Input: part model. Units: mm. Frame: model coordinates. Face numbers are marked on the shaded views. A direction names the side the tool comes from. Coordinates: 2 decimals unless noted, no trailing zeros. Write each loop counter-clockwise with the first axis right and the second up, starting at its lowest first coordinate (ties: lowest second). Pieces come first, ordered by that corner, then holes.
1) Section query D-D (x = -35). Output: boundary loops of the cut face in (y, z).
2) Draft query along X for the marked faces 4, 5, 6 and 7. Return one class per face: pulls with the +X half, pulls with the -X half, needs draft (parallel to the pull), parting line crosses it, or undercut.
3) Section query A-A (z = -18). Output: boundary loops of the cut face in (x, y).
4) Line query: L1, parallel to Z at x = -35, y = -13; L2, parallel to Y at x = -32, z = -43; L3, parallel to X at y = -11.5, z = -32. Output: solid intervals per line, ascending.
5) Pin query (flat end, axial travel): pin 1 Ø12 at (y, z) = (11.5, -42.5) entering from -X; pin 2 Ø20 at (x, y) = (-25.5, -6) entering from -Z; pin 3 Ø4 at (x, y) = (2.5, -11) entering from -Z. Return the tip coordinate at first contact, or that it passes through.
6) Set-up query: the marked faces 1, 2 and 3. Return all of +Z, -Z, +X, -X, +Y, -Y with unobstructed straight access to the full face (end or side cutting, diameter ignored); none if empty.
7) Section query B-B (x = 24). Output: boundary loops of the cut face in (y, z).
8) Section query C-C (z = -39). Output: boundary loops of the cut face in (x, y), then the cut area to 3 significant figures.
from build123d import *

# Parameters (mm, degrees)
SKETCH2_R           = 20
BOSS_EXTRUDE1_DEPTH = 8
CUT_EXTRUDE2_DEPTH  = 65.319514924
BOSS_EXTRUDE2_DEPTH = 12
SKETCH6_R           = 10
CUT_EXTRUDE3_DEPTH  = 91.647669578
FILLET2_R           = 1.2
FILLET3_R           = 1.2


with BuildPart() as part:
    # Sketch2 → Boss-Extrude1 (new, symmetric)
    with BuildSketch(Plane.XY):
        with BuildLine():
            Line((39, 20), (-59, 20))
            Line((-59, 20), (-59, -20))
            Line((-59, -20), (39, -20))
            ThreePointArc((39, -20), (19, 0), (39, 20))
        make_face()
        with Locations((39, 0)):
            Circle(SKETCH2_R)
    extrude(amount=BOSS_EXTRUDE1_DEPTH, both=True)

    # Sketch3 → Cut-Extrude2 (cut, through all)
    with BuildSketch(Plane.XY.offset(8)):
        with BuildLine():
            ThreePointArc((14.284953176, 0), (11.941807426, 5.656854249), (6.284953176, 8))
            Line((6.284953176, 8), (6.284953176, -8))
            ThreePointArc((6.284953176, -8), (11.941807426, -5.656854249), (14.284953176, 0))
        make_face()
        with BuildLine():
            Line((6.284953176, -8), (6.284953176, 8))
            ThreePointArc((6.284953176, 8), (-1.715046824, 0), (6.284953176, -8))
        make_face()
        with BuildLine():
            Line((30.284953176, 8), (6.284953176, 8))
            ThreePointArc((6.284953176, 8), (11.941807426, 5.656854249), (14.284953176, 0))
            ThreePointArc((14.284953176, 0), (11.941807426, -5.656854249), (6.284953176, -8))
            Line((6.284953176, -8), (30.284953176, -8))
            ThreePointArc((30.284953176, -8), (22.284953176, 0), (30.284953176, 8))
        make_face()
        with BuildLine():
            ThreePointArc((38.284953176, 0), (35.941807426, 5.656854249), (30.284953176, 8))
            Line((30.284953176, 8), (30.284953176, -8))
            ThreePointArc((30.284953176, -8), (35.941807426, -5.656854249), (38.284953176, 0))
        make_face()
        with BuildLine():
            Line((30.284953176, -8), (30.284953176, 8))
            ThreePointArc((30.284953176, 8), (22.284953176, 0), (30.284953176, -8))
        make_face()
    extrude(amount=-CUT_EXTRUDE2_DEPTH, mode=Mode.SUBTRACT)

    # Sketch5 → Boss-Extrude2 (add)
    with BuildSketch(Plane(origin=(0, 20, 0), x_dir=(1, 0, 0), z_dir=(0, 1, 0))):
        with BuildLine():
            ThreePointArc((-59, 32), (-51.970562748, 15.029437252), (-35, 8))
            ThreePointArc((-35, 8), (-18.029437252, 15.029437252), (-11, 32))
            Line((-11, 32), (-59, 32))
        make_face()
        with BuildLine():
            ThreePointArc((-11, 32), (-35, 56), (-59, 32))
            Line((-59, 32), (-11, 32))
        make_face()
        with BuildLine():
            Line((-59, 32), (-59, 8))
            Line((-59, 8), (-35, 8))
            ThreePointArc((-35, 8), (-51.970562748, 15.029437252), (-59, 32))
        make_face()
        with BuildLine():
            ThreePointArc((-11, 32), (-18.029437252, 15.029437252), (-35, 8))
            Line((-35, 8), (-11, 8))
            Line((-11, 8), (-11, 32))
        make_face()
    boss_extrude2 = extrude(amount=-BOSS_EXTRUDE2_DEPTH)

    # Sketch6 → Cut-Extrude3 (cut, through all)
    with BuildSketch(Plane(origin=(0, 20, 0), x_dir=(1, 0, 0), z_dir=(0, 1, 0))):
        with Locations(Location((-35, 32, 0), (0, 0, 180))):
            Circle(SKETCH6_R)
    cut_extrude3 = extrude(amount=-CUT_EXTRUDE3_DEPTH, mode=Mode.SUBTRACT)

    # Mirror1: Boss-Extrude2, Cut-Extrude3 across plane
    add(boss_extrude2.mirror(Plane.ZX))
    add(cut_extrude3.mirror(Plane.ZX), mode=Mode.SUBTRACT)

    # Fillet2
    fillet2_edges = [part.edges().sort_by_distance(p)[0] for p in [
        (-11, 14, -8),
    ]]
    fillet(fillet2_edges, radius=FILLET2_R)

    # Fillet3
    fillet3_edges = [part.edges().sort_by_distance(p)[0] for p in [
        (-11, -14, -8),
    ]]
    fillet(fillet3_edges, radius=FILLET3_R)


solid = part.part
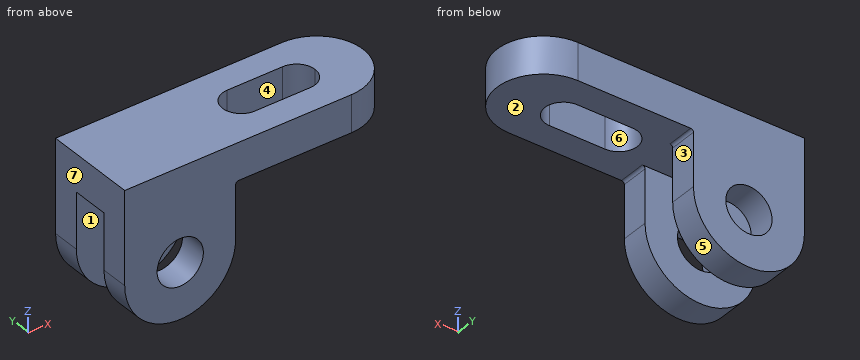
Answer:
1. outline: (-20, -56) - (-8, -56) - (-8, -42) - (-20, -42) - close; (-20, -22) - (-8, -22) - (-8, -8) - (8, -8) - (8, -22) - (20, -22) - (20, 8) - (-20, 8) - close; (8, -56) - (20, -56) - (20, -42) - (8, -42) - close
2. face 4: undercut
2. face 5: parting line crosses it
2. face 6: undercut
2. face 7: pulls with the -X half
3. outline: (-59, -20) - (-11, -20) - (-11, -8) - (-59, -8) - close; (-59, 8) - (-11, 8) - (-11, 20) - (-59, 20) - close
4. L1: z = -56 to -42, -22 to 8
4. L2: y = -20 to -8, 8 to 20
4. L3: x = -59 to -45, -25 to -11
5. pin 1: stops at x = -58.57
5. pin 2: stops at z = -56
5. pin 3: stops at z = -8
6. face 1: -Z, +X, -X
6. face 2: -Z, +X
6. face 3: -Z, +X, +Y, -Y
7. outline: (-20, -8) - (-8, -8) - (-8, 8) - (-20, 8) - close; (8, -8) - (20, -8) - (20, 8) - (8, 8) - close
8. outline: (-57.96, -20) - (-42.14, -20) - (-42.14, -8) - (-57.96, -8) - close; (-57.96, 8) - (-42.14, 8) - (-42.14, 20) - (-57.96, 20) - close; (-27.86, -20) - (-12.04, -20) - (-12.04, -8) - (-27.86, -8) - close; (-27.86, 8) - (-12.04, 8) - (-12.04, 20) - (-27.86, 20) - close
8. area: 759 mm2
